Source: CAD feature listing. Evaluate the final solid. Frame: model axes, mm. A direction names the side the tool comes from. Round coordinates to 2 decimals unless told otherwise and drop trailing zeros. Order: outer loops, then holes, each group sorted by start corner. A loop starts at its lowest first (then second) coordinate and runs counter-clockwise, first axis right, second up. Notation, with made-up numbers: (38.25, 35.5) - (86.25, 35.5) arc R5 cw to (86.25, 40.5) - close; hole circle Ø7 at (13, 56). An arc over 180 degrees is marked (long way). Use one line per item in the form item = value. Start each with the question number.
Q1. Set-up query: faces 5 (the flat face through (27.68, 0, 21)), 6 (the flat face through (0, -25.6, 2)), 7 (the cylindrical face through (-25.75, -25.63, 8.92)), 8 (the cylindrical face through (21.89, 6.89, 41.05)), 9 (the cylindrical face through (-20.345, 21.021, 1.972)). Return all of +Z, -Z, +X, -X, +Y, -Y with unobstructed straight access to the full face (end or side cutting, diameter ignored); none if empty.
Q2. Draft query along X for faces 1 (the flat face through (4.5, -27, 2)), 2 (the flat face through (0, 0, 41.3)), 3 (the flat face through (27.8, 0, 9)), 4 (the cylindrical face through (-20.345, -21.979, 1.972)). Return one class per face: released by +X, released by -X, zero draft, split by the parting line, or undercut.
Q3. Cut plane B-B, the plane z = 30. Return the cut outline in (x, y), and give its area (3 significant figures).
Q4. Pin query (flat end, axial travel): pin 1 Ø2 at (x, y) = (-21.5, -21.5) entering from -Z; pin 2 Ø2.5 at (y, z) = (8, 19.5) entering from +X; pin 3 Ø1.1 at (y, z) = (-26.5, 2) entering from -X. Return the tip coordinate at first contact, or that it passes through.
Q5. Ray query, line 1 (X direction, y = 0, z = 41.2); line 2 (Y direction, x = 21.5, z = 2.7); line 3 (Y direction, x = -21.5, z = 22.8). Return the intervals inside material, ascending. Write a range as [from, to].
from build123d import *

# Parameters (mm, degrees)
BASE_HOUSING_DEPTH                     = 18.1
UPPER_START                            = 18
UPPER_HOUSING_RIM_DEPTH                = 5.1
OPTICAL_START                          = 23
OPTICAL_ENCLOSURE_PROFILE_R            = 25
OPTICAL_ENCLOSURE_DEPTH                = 15.1
TAPERED_START                          = 38
TAPERED_COVER_PROFILE_R                = 25
TAPERED_COVER_DEPTH                    = 2.8
TAPERED_COVER_TAPER                    = 34.159694546
COVER_START                            = 40.7
COVER_DISK_PROFILE_R                   = 22.95
COVER_DISK_DEPTH                       = 0.6
FOUR_START                             = -0.05
FOUR_M2_5_MOUNTING_POSITIONS_PROFILE_R = 1.25
FOUR_M2_5_MOUNTING_POSITIONS_DEPTH     = 4.05
UPPER_START_2                          = 22.3
UPPER_RECESSES_PROFILE_R               = 1.75
UPPER_RECESSES_DEPTH                   = 1
CABLE_START                            = -0.05
CABLE_OUTLET_RECESS_PROFILE_W          = 9
CABLE_OUTLET_RECESS_PROFILE_H          = 2.4
CABLE_OUTLET_RECESS_DEPTH              = 3.35
COVER_START_2                          = 41.1
COVER_GROOVE_PROFILE_R                 = 12.7
COVER_GROOVE_PROFILE_R_2               = 12.25
COVER_GROOVE_DEPTH                     = 0.4


with BuildPart() as part:
    # Base housing profile → Base housing (new body)
    with BuildSketch(Plane.XY):
        with BuildLine():
            Line((-20.6, -27.8), (20.6, -27.8))
            ThreePointArc((20.6, -27.8), (25.691168825, -25.691168825), (27.8, -20.6))
            Line((27.8, -20.6), (27.8, 20.6))
            ThreePointArc((27.8, 20.6), (25.691168825, 25.691168825), (20.6, 27.8))
            Line((20.6, 27.8), (-20.6, 27.8))
            ThreePointArc((-20.6, 27.8), (-25.691168825, 25.691168825), (-27.8, 20.6))
            Line((-27.8, 20.6), (-27.8, -20.6))
            ThreePointArc((-27.8, -20.6), (-25.691168825, -25.691168825), (-20.6, -27.8))
        make_face()
    extrude(amount=BASE_HOUSING_DEPTH)

    # Upper housing rim profile → Upper housing rim (add)
    with BuildSketch(Plane.XY.offset(UPPER_START)):
        with BuildLine():
            Line((-20.6, -27.68), (20.6, -27.68))
            ThreePointArc((20.6, -27.68), (25.606316011, -25.606316011), (27.68, -20.6))
            Line((27.68, -20.6), (27.68, 20.6))
            ThreePointArc((27.68, 20.6), (25.606316011, 25.606316011), (20.6, 27.68))
            Line((20.6, 27.68), (-20.6, 27.68))
            ThreePointArc((-20.6, 27.68), (-25.606316011, 25.606316011), (-27.68, 20.6))
            Line((-27.68, 20.6), (-27.68, -20.6))
            ThreePointArc((-27.68, -20.6), (-25.606316011, -25.606316011), (-20.6, -27.68))
        make_face()
    extrude(amount=UPPER_HOUSING_RIM_DEPTH)

    # Optical enclosure profile → Optical enclosure (add)
    with BuildSketch(Plane.XY.offset(OPTICAL_START)):
        Circle(OPTICAL_ENCLOSURE_PROFILE_R)
    extrude(amount=OPTICAL_ENCLOSURE_DEPTH)

    # Tapered cover profile → Tapered cover (add)
    with BuildSketch(Plane.XY.offset(TAPERED_START)):
        Circle(TAPERED_COVER_PROFILE_R)
    extrude(amount=TAPERED_COVER_DEPTH, taper=TAPERED_COVER_TAPER)

    # Cover disk profile → Cover disk (add)
    with BuildSketch(Plane.XY.offset(COVER_START)):
        Circle(COVER_DISK_PROFILE_R)
    extrude(amount=COVER_DISK_DEPTH)

    # Four M2.5 mounting positions profile → Four M2.5 mounting positions (cut)
    with BuildSketch(Plane.XY.offset(FOUR_START)):
        with Locations((-21.5, -21.5)):
            Circle(FOUR_M2_5_MOUNTING_POSITIONS_PROFILE_R)
        with Locations((-21.5, 21.5)):
            Circle(FOUR_M2_5_MOUNTING_POSITIONS_PROFILE_R)
        with Locations((21.5, -21.5)):
            Circle(FOUR_M2_5_MOUNTING_POSITIONS_PROFILE_R)
        with Locations((21.5, 21.5)):
            Circle(FOUR_M2_5_MOUNTING_POSITIONS_PROFILE_R)
    extrude(amount=FOUR_M2_5_MOUNTING_POSITIONS_DEPTH, mode=Mode.SUBTRACT)

    # Upper recesses profile → Upper recesses (cut)
    with BuildSketch(Plane.XY.offset(UPPER_START_2)):
        with Locations((-21.5, -21.5)):
            Circle(UPPER_RECESSES_PROFILE_R)
        with Locations((-21.5, 21.5)):
            Circle(UPPER_RECESSES_PROFILE_R)
        with Locations((21.5, -21.5)):
            Circle(UPPER_RECESSES_PROFILE_R)
        with Locations((21.5, 21.5)):
            Circle(UPPER_RECESSES_PROFILE_R)
    extrude(amount=UPPER_RECESSES_DEPTH, mode=Mode.SUBTRACT)

    # Cable outlet recess profile → Cable outlet recess (cut)
    with BuildSketch(Plane.XY.offset(CABLE_START)):
        with Locations((0, -26.8)):
            Rectangle(CABLE_OUTLET_RECESS_PROFILE_W, CABLE_OUTLET_RECESS_PROFILE_H)
    extrude(amount=CABLE_OUTLET_RECESS_DEPTH, mode=Mode.SUBTRACT)

    # Cover groove profile → Cover groove (cut)
    with BuildSketch(Plane.XY.offset(COVER_START_2)):
        Circle(COVER_GROOVE_PROFILE_R)
        Circle(COVER_GROOVE_PROFILE_R_2, mode=Mode.SUBTRACT)
    extrude(amount=COVER_GROOVE_DEPTH, mode=Mode.SUBTRACT)


solid = part.part
Completed:
q1.face_5 = +Z, +X, +Y, -Y
q1.face_6 = -Z, -Y
q1.face_7 = +Z, -Z, -X, -Y
q1.face_8 = +Z
q1.face_9 = -Z
q2.face_1 = undercut
q2.face_2 = zero draft
q2.face_3 = released by +X
q2.face_4 = undercut
q3.outline = circle Ø50 at (0, 0)
q3.area = 1,960 mm2
q4.pin_1 = 4
q4.pin_2 = 27.68
q4.pin_3 = -25.42
q5.line_1 = [-22.95, -12.7], [-12.25, 12.25], [12.7, 22.95]
q5.line_2 = [-27.74, -22.75], [-20.25, 20.25], [22.75, 27.74]
q5.line_3 = [-27.62, -23.25], [-19.75, 19.75], [23.25, 27.62]
